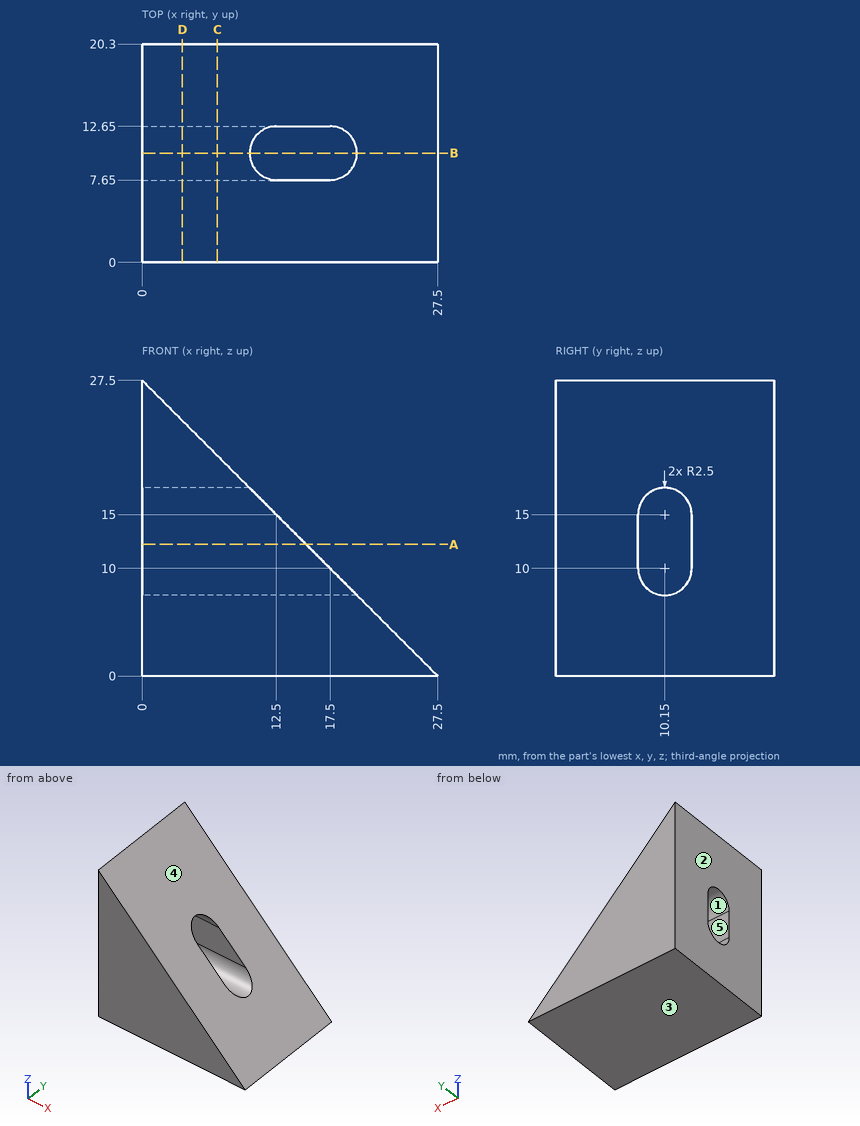
Source: three-view drawing plus pictorial views. Frame: mm from the lowest corner of the part. A direction names the side the tool comes from. Round coordinates to 2 decimals unless told otherwise and drop trailing zeros. Write each loop counter-clockwise with the first axis right and the second up, starting at its lowest first coordinate (ties: lowest second). Pieces come first, ordered by that corner, then holes. Notation, with made-up numbers: M 87.25,48 L 122.25,48 A16 ccw 122.25,53 Z; hole C 51.25,0 d6. An arc over 180 degrees is marked long. Write item = value, one per line.
Item 1: Section query B-B on y = 10.15. Return loops of the section in (x, z).
Findings:
outline = M 0,0 L 27.5,0 L 20,7.5 L 0,7.5 Z; M 0,17.5 L 10,17.5 L 0,27.5 Z
Item 2: Section query D-D on x = 3.75. Return loops of the section in (y, z), then the cut area to 3 significant figures.
Findings:
outline = M 0,0 L 20.3,0 L 20.3,23.75 L 0,23.75 Z; hole M 7.65,10 A2.5 ccw 12.65,10 L 12.65,15 A2.5 ccw 7.65,15 Z
area = 437 mm^2
Item 3: Pin query (flat end, axial travel): P1, Ø1, axis at x = 24.5, y = 15, coming from the +Z side; P2, Ø6, axis at x = 7, y = 2.5, coming from the +Z side; P3, Ø6, axis at y = 13.5, z = 10, coming from the +X side. Return the tip coordinate at first contact, or that it passes through.
Findings:
P1 = 3.5
P2 = 23.5
P3 = 20.5
Item 4: Pull-direction query (Z, two-part tool) for the marked faces 1, 2 and 3; classes: pulls with the +Z half, pulls with the -Z half, needs draft (parallel to the pull), parting line crosses it, or undercut.
Findings:
face_1 = undercut
face_2 = needs draft
face_3 = pulls with the -Z half
Item 5: Section query A-A on z = 12.25. Return loops of the section in (x, y).
Findings:
outline = M 0,0 L 15.25,0 L 15.25,7.65 L 0,7.65 Z; M 0,12.65 L 15.25,12.65 L 15.25,20.3 L 0,20.3 Z
Item 6: Section query C-C on x = 7. Return loops of the section in (y, z).
Findings:
outline = M 0,0 L 20.3,0 L 20.3,20.5 L 0,20.5 Z; hole M 7.65,10 A2.5 ccw 12.65,10 L 12.65,15 A2.5 ccw 7.65,15 Z
Item 7: Access query for the marked faces 4 and 5. Directions: +Z, -Z, +X, -X, +Y, -Y. A direction counts if a zero-diameter tool reaches every point of the face in a straight line with its end or side. Return the directions, or none.
Findings:
face_4 = +Z, +X, +Y, -Y
face_5 = +X, -X
Item 8: Material intervals for line 1 along Y through (x, z) = (7.5, 17.25); line 2 along Z through (x, y) = (4.75, 9.25); line 3 along Y through (x, z) = (3.5, 16.75), sorted ascending. Write a range as [from, to].
Findings:
line_1 = [0, 9.06], [11.24, 20.3]
line_2 = [0, 7.67], [17.33, 22.75]
line_3 = [0, 8.36], [11.94, 20.3]
